Input: part model. Units: mm. Frame: model coordinates. A direction names the side the tool comes from. Round coordinates to 2 decimals unless told otherwise and drop trailing zeros. Write each loop counter-clockwise with the first axis right and the second up, starting at its lowest first coordinate (ties: lowest second). Pieces come first, ordered by that corner, then holes. Notation, with made-up numbers: (63, -22) - (70, -22) arc R20 cw to (70, 16) - close; hole circle Ø3 at (21, 64). An arc over 180 degrees is marked (long way). One line per item, written item: value. Start each with the question number.
```python
from build123d import *

# Parameters (mm, degrees)
F3_DEPTH     = 5
F4_T4_ANGLE  = 270.6670948428
F4_S5_R      = 2
F4_T6_DEPTH  = 5
F4_T10_ANGLE = 262.8807253971
F4_S11_R     = 2
F4_T12_DEPTH = 5
F5_SIZE      = 1
F6_R         = 1
F7_R         = 0.49999
F8_R         = 0.5
F9_W         = 20.6344220787
F9_H         = 19.8933202773
F9_R         = 5
F10_DEPTH    = 5
F11_R        = 2.8
F12_DEPTH    = 6.4


# Not quite as in the source:
# - a fillet or chamfer that OpenCascade refuses, or shapes differently, is made with other operations: its cross-section is extruded or revolved along the edge and cut away or added
# - a fillet or chamfer is up to 0.001 mm smaller than in the source, because OpenCascade refuses the exact size


with BuildPart() as f1:
    # F0 (on Right) → F1 (revolve)
    with BuildSketch(Plane.YZ):
        Polygon((-6, 0), (0, 0), (0, 12), (-1, 12), (-1, 16), (-1, 19), (-2, 19), (-2.5, 19), (-2.5, 16), (-2, 16), (-2, 12), (-6, 12), align=None)
    revolve(axis=Axis((0, 0, 6), (0, 0, -1)))

    # F2 (on face) → F3 (cut)
    with BuildSketch(Plane.XY.offset(19)):
        with BuildLine():
            Line((-0.8067003414, 0.5909607086), (-2.4291491187, 0.5909607086))
            ThreePointArc((-2.4291491187, 0.5909607086), (-2.4985623215, -0.0847721969), (-2.3835084063, -0.75424643))
            Line((-2.3835084063, -0.75424643), (-0.6565914428, -0.75424643))
            ThreePointArc((-0.6565914428, -0.75424643), (-0.993831612, -0.1108996261), (-0.8067003414, 0.5909607086))
        make_face()
        with BuildLine():
            ThreePointArc((1, 0), (0.9504473529, 0.3108855566), (0.8067003414, 0.5909607086))
            Line((0.8067003414, 0.5909607086), (-0.8067003414, 0.5909607086))
            ThreePointArc((-0.8067003414, 0.5909607086), (-0.993831612, -0.1108996261), (-0.6565914428, -0.75424643))
            Line((-0.6565914428, -0.75424643), (0.6565914428, -0.75424643))
            ThreePointArc((0.6565914428, -0.75424643), (0.9101075329, -0.4143721499), (1, 0))
        make_face()
        with BuildLine():
            ThreePointArc((2.5, 0), (2.482224083, 0.2975963737), (2.4291491187, 0.5909607086))
            Line((2.4291491187, 0.5909607086), (0.8067003414, 0.5909607086))
            ThreePointArc((0.8067003414, 0.5909607086), (0.9504473529, 0.3108855566), (1, 0))
            ThreePointArc((1, 0), (0.9101075329, -0.4143721499), (0.6565914428, -0.75424643))
            Line((0.6565914428, -0.75424643), (2.3835084063, -0.75424643))
            ThreePointArc((2.3835084063, -0.75424643), (2.4707054676, -0.38159467), (2.5, 0))
        make_face()
    extrude(amount=-F3_DEPTH, mode=Mode.SUBTRACT)

    # F4: chamfer of 1 on 2 edges, made by hand


with BuildPart() as f4_tool2:
    # F4_s3 → F4_t4 (revolve)
    with BuildSketch(Plane(origin=(0, 0, 0), x_dir=(0, 0, 1), z_dir=(0.7112111987, -0.7029784, 0))):
        Polygon((17, 2.5), (16, 1.5), (16, 2.5), align=None)
    revolve(axis=Axis((0, 0, 16), (0, 0, -1)), revolution_arc=F4_T4_ANGLE)

    # F4_s5 → F4_t6 (cut, symmetric)
    with BuildSketch(Plane.XY.offset(16.5)):
        Circle(F4_S5_R)
    extrude(amount=F4_T6_DEPTH, both=True, mode=Mode.SUBTRACT)


with BuildPart() as f1_1:
    add(f1.part)

    # F4_t1: cut F4_tool2
    add(f4_tool2.part, mode=Mode.SUBTRACT)


with BuildPart() as f4_tool8:
    # F4_s9 → F4_t10 (revolve)
    with BuildSketch(Plane(origin=(0, 0, 0), x_dir=(0, 0, 1), z_dir=(-0.6618401259, 0.7496450145, 0))):
        Polygon((17, 2.5), (16, 1.5), (16, 2.5), align=None)
    revolve(axis=Axis((0, 0, 16), (0, 0, -1)), revolution_arc=F4_T10_ANGLE)

    # F4_s11 → F4_t12 (cut, symmetric)
    with BuildSketch(Plane.XY.offset(16.5)):
        Circle(F4_S11_R)
    extrude(amount=F4_T12_DEPTH, both=True, mode=Mode.SUBTRACT)


with BuildPart() as f1_2:
    add(f1_1.part)

    # F4_t7: cut F4_tool8
    add(f4_tool8.part, mode=Mode.SUBTRACT)

    # F5
    f5_edges = [f1_2.edges().sort_by_distance(p)[0] for p in [
        (0, 6, 0),
    ]]
    chamfer(f5_edges, length=F5_SIZE)

    # F6
    f6_edges = [f1_2.edges().sort_by_distance(p)[0] for p in [
        (0, 1, 19),
        (-0.350538, -0.936549, 19),
        (0.350538, -0.936549, 19),
    ]]
    fillet(f6_edges, radius=F6_R)

    # F7 (radius 0.5 in the source; OpenCascade refuses exactly that, so slightly less here)
    f7_edges = [f1_2.edges().sort_by_distance(p)[0] for p in [
        (0, -2.5, 19),
        (0, 2.5, 19),
    ]]
    fillet(f7_edges, radius=F7_R)

    # F8
    f8_edges = [f1_2.edges().sort_by_distance(p)[0] for p in [
        (-1.254459, -0.754246, 14),
        (1.254459, -0.754246, 14),
        (-1.358699, 0.590961, 14),
        (1.358699, 0.590961, 14),
    ]]
    fillet(f8_edges, radius=F8_R)

    # F9 (on face) → F10 (cut)
    with BuildSketch(Plane(origin=(0, 0, 0), x_dir=(1, 0, 0), z_dir=(0, 0, -1))):
        with Locations((1.0028546676, -0.4471866414)):
            Rectangle(F9_W, F9_H)
        Circle(F9_R, mode=Mode.SUBTRACT)
        Circle(F9_R)
    extrude(amount=-F10_DEPTH, mode=Mode.SUBTRACT)

    # F11 (on face) → F12 (cut)
    with BuildSketch(Plane(origin=(0, 0, 5), x_dir=(1, 0, 0), z_dir=(0, 0, -1))):
        Circle(F11_R)
    extrude(amount=-F12_DEPTH, mode=Mode.SUBTRACT)


solid = f1_2.part
```
Q1. Access query for faces 1 (the cylindrical face through (0, 2.5, 17.7)), 2 (the flat face through (1, 0.591, 17)), 3 (the cylindrical face through (0, 1, 14)), 4 (the cylindrical face through (0, -2.5, 17.7)), 5 (the cylindrical face through (-2.8, -0.1, 8.2)). Directions: +Z, -Z, +X, -X, +Y, -Y. A direction counts if a zero-diameter tool reaches every point of the face in a straight line with its end or side. Return the directions, or none.
Q2. Material intervals for probe 1 along Y at (x, z) = (0.25, 12.75); probe 2 along Y at (x, z) = (0, 6.75), sorted ascending. Write a range as from..to.
Q3. Contact query for flat-ended pins moving along their axis: pin 1 Ø1.3 at (x, z) = (-1.5, 17.5) entering from -Y; pin 2 Ø1.5 at (y, z) = (1.5, 7.5) entering from +X; pin 3 Ø3 at (x, y) = (0, 0) entering from +Z. Output: stop coordinate, or through.
Q4. Cut plane A-A, the plane z = 17.5. Output: boundary loops of the cut face in (x, y), and give its area (3 significant figures).
Q5. Cut plane B-B, the plane z = 10.25. Output: boundary loops of the cut face in (x, y), and give its area (3 significant figures).
Q6. Cut plane D-D, the plane x = 5.25. Output: boundary loops of the cut face in (y, z).
Q7. Pull-direction query (Z, two-part tool) for faces 6 (the conical face through (0.04, -2.14, 16.64)), 7 (the flat face through (0, 0, 11.4)), 8 (the cylindrical face through (0, 6, 8)); classes: pulls with the +Z half, pulls with the -Z half, needs draft (parallel to the pull), parting line crosses it, or undercut.
Q8. Cut plane C-C, the plane y = -0.5. Output: boundary loops of the cut face in (x, z) (1 decimal), and give its area (3 significant figures).
A:
1. face 1: +Z, +Y
1. face 2: +Z, +X, -X
1. face 3: +Z
1. face 4: +Z, -Y
1. face 5: -Z
2. probe 1: y = -1.98..-0.97, 0.97..1.98
2. probe 2: y = -6..-2.8, 2.8..6
3. pin 1: stops at y = -2.35
3. pin 2: stops at x = 5.95
3. pin 3: stops at z = 18.87
4. outline: (-2.43, 0.59) - (-0.81, 0.59) arc R1 cw to (0.81, 0.59) - (2.43, 0.59) arc R2.5 ccw to start; (-2.38, -0.75) arc R2.5 ccw to (2.38, -0.75) - (0.66, -0.75) arc R1 cw to (-0.66, -0.75) - close
4. area: 12.3 mm²
5. outline: circle Ø12 at (0, 0); hole circle Ø5.6 at (0, 0)
5. area: 88.5 mm²
6. outline: (-2.9, 5) - (2.9, 5) - (2.9, 12) - (-2.9, 12) - close
7. face 6: undercut
7. face 7: pulls with the -Z half
7. face 8: needs draft
8. outline: (-6, 5) - (-2.8, 5) - (-2.8, 11.4) - (2.8, 11.4) - (2.8, 5) - (6, 5) - (6, 12) - (1.9, 12) - (1.9, 14.1) - (0.9, 14.1) - (0.9, 12) - (-0.9, 12) - (-0.9, 14.1) - (-1.9, 14.1) - (-1.9, 12) - (-6, 12) - close
8. area: 52.9 mm²
